Could you check a few things on this model? Use its own coordinates, in mm. A direction names the side the tool comes from. Give positions to 0.01 mm unless a question says otherwise; leave off trailing zeros. Write each loop counter-clockwise with the first axis right and the second up, starting at its lowest first coordinate (ties: lowest second). Pieces come first, ordered by that corner, then holes. Notation, with made-up numbers: (0, -40) - (48, -40) arc R3 ccw to (48, -35) - close; hole circle Ø5 at (10, 19.5). An arc over 180 degrees is marked (long way). Use one line per item in the form item = value.
```python
from build123d import *

# Parameters (mm, degrees)
F0_W     = 53
F0_H     = 35
F1_DEPTH = 4
F2_R     = 1.4
F3_DEPTH = 25
F4_W     = 7.5
F4_H     = 6.995946
F4_R     = 1.4
F4_H_2   = 9
F5_DEPTH = 7


with BuildPart() as f1:
    # F0 (on Top) → F1 (new body)
    with BuildSketch(Plane.XY):
        with Locations((26.5, 17.5)):
            Rectangle(F0_W, F0_H)
        with BuildLine():
            ThreePointArc((4.484879, 6.248995), (2.734879, 7.998995), (4.484879, 9.748995))
            Line((4.484879, 9.748995), (9.484879, 9.748995))
            ThreePointArc((9.484879, 9.748995), (11.234879, 7.998995), (9.484879, 6.248995))
            Line((9.484879, 6.248995), (4.484879, 6.248995))
        make_face(mode=Mode.SUBTRACT)
        with BuildLine():
            ThreePointArc((44.676833, 6.244954), (42.926833, 7.994954), (44.676833, 9.744954))
            Line((44.676833, 9.744954), (49.676833, 9.744954))
            ThreePointArc((49.676833, 9.744954), (51.426833, 7.994954), (49.676833, 6.244954))
            Line((49.676833, 6.244954), (44.676833, 6.244954))
        make_face(mode=Mode.SUBTRACT)
        with BuildLine():
            ThreePointArc((4.5, 20.25), (2.75, 22), (4.5, 23.75))
            Line((4.5, 23.75), (9.5, 23.75))
            ThreePointArc((9.5, 23.75), (11.25, 22), (9.5, 20.25))
            Line((9.5, 20.25), (4.5, 20.25))
        make_face(mode=Mode.SUBTRACT)
        with BuildLine():
            ThreePointArc((44.675402, 20.246368), (42.925402, 21.996368), (44.675402, 23.746368))
            Line((44.675402, 23.746368), (49.675402, 23.746368))
            ThreePointArc((49.675402, 23.746368), (51.425402, 21.996368), (49.675402, 20.246368))
            Line((49.675402, 20.246368), (44.675402, 20.246368))
        make_face(mode=Mode.SUBTRACT)
    extrude(amount=F1_DEPTH)

    # F2 (on face) → F3 (cut)
    with BuildSketch(Plane.XY.offset(4)):
        with Locations((4.094722, 31.5)):
            Circle(F2_R)
        with Locations((4.306453, 12.5)):
            Circle(F2_R)
    extrude(amount=-F3_DEPTH, mode=Mode.SUBTRACT)

    # F4 (on face) → F5 (join)
    with BuildSketch(Plane.XY.offset(4)):
        with Locations((3.75, 14.002027)):
            Rectangle(F4_W, F4_H)
        with Locations((4.306453, 12.5)):
            Circle(F4_R, mode=Mode.SUBTRACT)
        with Locations((3.75, 30.5)):
            Rectangle(F4_W, F4_H_2)
        with Locations((4.094722, 31.5)):
            Circle(F4_R, mode=Mode.SUBTRACT)
    extrude(amount=F5_DEPTH)


solid = f1.part
```
1. Imagine slicing it at D-D, the plane y = 31.5. List the corners of the cut face in (x, z) for me, and give its area (3 significant figures).
Response values:
outline = (0, 0) - (2.69, 0) - (2.69, 11) - (0, 11) - close; (5.49, 0) - (53, 0) - (53, 4) - (7.5, 4) - (7.5, 11) - (5.49, 11) - close
area = 234 mm²
2. If we mould it in two halves opening along X, with no side actions, what happens to faces 4 (the face through (47, 20.246, 2)), 5 (the face through (53, 17, 2)), 6 (the face through (26, 0, 2))? For each: pulls with the +X half, pulls with the -X half, needs draft (parallel to the pull), parting line crosses it, or undercut.
Response values:
face_4 = undercut
face_5 = pulls with the +X half
face_6 = needs draft
3. Which directions (+Z, -Z, +X, -X, +Y, -Y) give clear straight access to the entire face, cutting with the end or side of a thin tool? Please do faces 1 (the face through (7, 9.749, 2)), 2 (the face through (4, 26, 7)), 3 (the face through (7.5, 14, 7)).
Response values:
face_1 = +Z, -Z
face_2 = +Z, +X, -X
face_3 = +Z, +X, +Y, -Y
4. Imagine slicing it at C-C, the plane x = 49. List the corners of the cut face in (y, z) for me.
Response values:
outline = (0, 0) - (6.24, 0) - (6.24, 4) - (0, 4) - close; (9.74, 0) - (20.25, 0) - (20.25, 4) - (9.74, 4) - close; (23.75, 0) - (35, 0) - (35, 4) - (23.75, 4) - close
5. Imagine slicing it at A-A, the plane z = 5.75. List the corners of the cut face in (x, y) for me, and give its area (3 significant figures).
Response values:
outline = (0, 10.5) - (7.5, 10.5) - (7.5, 17.5) - (0, 17.5) - close; (0, 26) - (7.5, 26) - (7.5, 35) - (0, 35) - close; hole circle Ø2.8 at (4.09, 31.5); hole circle Ø2.8 at (4.31, 12.5)
area = 108 mm²
6. For pin 1 (2 mm diameter, centred on x = 4.5, z = 7.5, fed in from -Y); pin 2 (6 mm diameter, centred on x = 33, y = 23, fed in from +Z); pin 3 (3 mm diameter, centred on x = 38.5, z = 7, fed in from -Y), each with a flat end and sliding along its axis, tell me the tip position at first contact or that it passes through.
Response values:
pin_1 = 10.5
pin_2 = 4
pin_3 = through
7. Imagine slicing it at B-B, the plane y = 22. List the corners of the cut face in (x, z) for me, and give its area (3 significant figures).
Response values:
outline = (0, 0) - (2.75, 0) - (2.75, 4) - (0, 4) - close; (11.25, 0) - (42.93, 0) - (42.93, 4) - (11.25, 4) - close; (51.43, 0) - (53, 0) - (53, 4) - (51.43, 4) - close
area = 144 mm²
8. If I drill on line 1 (Y direction, x = 47, z = 3.5); line 2 (Y direction, x = 44, z = 2.75); line 3 (Z direction, x = 17, y = 9.5), over which ranges is the centre line in solid material (lowest first)? Write a range as from..to.
Response values:
line_1 = 0..6.24, 9.74..20.25, 23.75..35
line_2 = 0..6.38, 9.61..20.38, 23.61..35
line_3 = 0..4
